Here's how the part is built. I have some questions about the finished solid (model axes, mm). A direction names the side the tool comes from. Round coordinates to 2 decimals unless told otherwise and drop trailing zeros. Write each loop counter-clockwise with the first axis right and the second up, starting at its lowest first coordinate (ties: lowest second). Pieces come first, ordered by that corner, then holes. Notation, with made-up numbers: (-39, 30) -> (-22, 30) arc R6 ccw to (-22, 41) -> close; hole circle Ø7 at (85, -26.75). An arc over 180 degrees is marked (long way). Put each result on its own line as item: value. Start each with the question number.
1) If I drill on line 1 along X through (y, z) = (14.75, -7.5); line 2 along Z through (x, y) = (8.5, 11.5); line 3 along Z through (x, y) = (14, 6), over which ranges is the centre line in solid material (lowest first)? Write a range as [from, to].
2) I want a section at A-A, the plane z = -7. List the corners of the cut face in (x, y) for me.
3) We'd pull the mould along Z, two halves only. Please class faces 1 (the conical face through (3.18, 16.99, -3.24)), 2 (the conical face through (37.436, 16.986, -80.218)), 3 (the flat face through (0.947, 16.986, -40.345)), 4 (the conical face through (35.82, 16.99, -78.51)): released by +Z, released by -Z, zero draft, split by the parting line, or undercut.
4) I want a section at D-D, the plane y = 11. List the corners of the cut face in (x, z) for me, then the cut area to 4 significant figures.
5) Will these pins go through, and if not, where does the flat tip stop? P1, Ø0.9, axis at y = 11, z = -2, coming from the -X side; P2, Ø1.5, axis at x = 21, z = -2, coming from the +Y side; P3, Ø2, axis at y = 16.5, z = -79.5, coming from the +X side; P4, Ø3.5, axis at x = 8.5, z = -54, coming from the +Y side.
6) I want a section at C-C, the plane y = 15.25. List the corners of the cut face in (x, z) for me, then the cut area to 3 significant figures.
7) I want a section at B-B, the plane x = 30. List the corners of the cut face in (y, z) for me.
8) Which directions (+Z, -Z, +X, -X, +Y, -Y) give clear straight access to the entire face, cutting with the end or side of a thin tool? Please do faces 5 (the cylindrical face through (38.1, 8.6, -0.86)), 6 (the flat face through (11, 11, -1)), 7 (the flat face through (19, 14, -80)), 8 (the conical face through (37.5, 17, -1.6)), 9 (the flat face through (8.465, 16.986, -2.053)).
from build123d import *

# Parameters (mm, degrees)
SKETCH1_W                 = 39
SKETCH1_H                 = 81.75
BOSS_EXTRUDE1_DEPTH       = 3
SKETCH2_W                 = 39
SKETCH2_H                 = 81.75
SKETCH2_W_2               = 33
SKETCH2_H_2               = 75.75
BOSS_EXTRUDE2_DEPTH       = 15
SKETCH4_W                 = 17
SKETCH4_H                 = 3
CUT_EXTRUDE1_DEPTH        = 14
SKETCH4_3_W               = 12
SKETCH4_3_H               = 3
CUT_EXTRUDE2_DEPTH        = 4
FILLET1_R                 = 3
STANDOFFS1_GROOVE_DEPTH   = 2
STANDOFFS1_GROOVE_DRAFT   = -3
STANDOFFS1_GROOVE_2_DEPTH = 2
STANDOFFS1_GROOVE_2_DRAFT = -3
STANDOFFS2_GROOVE_DEPTH   = 2
STANDOFFS2_GROOVE_DRAFT   = -3
STANDOFFS2_GROOVE_2_DEPTH = 2
STANDOFFS2_GROOVE_2_DRAFT = -3
FILLET2_R                 = 2
CHAMFER1_SIZE             = 1


# Read off the part's stored shape, not the designer's step: Standoffs1-Groove, Standoffs2-Groove
with BuildPart() as part:
    # Sketch1 → Boss-Extrude1 (new body)
    with BuildSketch(Plane(origin=(0, 0, 0), x_dir=(1, 0, 0), z_dir=(0, 1, 0))):
        with Locations((19.5, 40.875)):
            Rectangle(SKETCH1_W, SKETCH1_H)
    extrude(amount=BOSS_EXTRUDE1_DEPTH)

    # Sketch2 → Boss-Extrude2 (add)
    with BuildSketch(Plane(origin=(0, 3, 0), x_dir=(1, 0, 0), z_dir=(0, 1, 0))):
        with Locations((19.5, 40.875)):
            Rectangle(SKETCH2_W, SKETCH2_H)
        with Locations((19.5, 40.875)):
            Rectangle(SKETCH2_W_2, SKETCH2_H_2, mode=Mode.SUBTRACT)
    extrude(amount=BOSS_EXTRUDE2_DEPTH)

    # Sketch4 → Cut-Extrude1 (cut)
    with BuildSketch(Plane(origin=(0, 18, 0), x_dir=(1, 0, 0), z_dir=(0, 1, 0))):
        with Locations((19.5, 1.5)):
            Rectangle(SKETCH4_W, SKETCH4_H)
    extrude(amount=-CUT_EXTRUDE1_DEPTH, mode=Mode.SUBTRACT)

    # Sketch4<3> → Cut-Extrude2 (cut)
    with BuildSketch(Plane(origin=(0, 18, 0), x_dir=(1, 0, 0), z_dir=(0, 1, 0))):
        with Locations((19.5, 80.25)):
            Rectangle(SKETCH4_3_W, SKETCH4_3_H)
    extrude(amount=-CUT_EXTRUDE2_DEPTH, mode=Mode.SUBTRACT)

    # Fillet1
    fillet1_edges = [part.edges().sort_by_distance(p)[0] for p in [
        (3, 10.5, -78.75),
        (3, 10.5, -3),
        (36, 10.5, -3),
        (36, 10.5, -78.75),
        (0, 9, -81.75),
        (39, 9, -81.75),
        (39, 9, 0),
        (0, 9, 0),
    ]]
    fillet(fillet1_edges, radius=FILLET1_R)


with BuildPart() as standoffs1_groove_tool:
    # Standoffs1-Groove outline → Standoffs1-Groove (with draft: the straight prism first)
    with BuildSketch(Plane(origin=(0, 16, 0), x_dir=(1, 0, 0), z_dir=(0, 1, 0))):
        with BuildLine():
            Line((11, 0.895184441), (3, 0.895184441))
            ThreePointArc((3, 0.895184441), (1.511670645, 1.511670645), (0.895184441, 3))
            Line((0.895184441, 3), (0.895184441, 78.75))
            ThreePointArc((0.895184441, 78.75), (1.511670645, 80.238329355), (3, 80.854815559))
            Line((3, 80.854815559), (13.5, 80.854815559))
            Line((13.5, 80.854815559), (13.5, 81.75))
            Line((13.5, 81.75), (3, 81.75))
            ThreePointArc((3, 81.75), (0.878679656, 80.871320344), (0, 78.75))
            Line((0, 78.75), (0, 3))
            ThreePointArc((0, 3), (0.878679656, 0.878679656), (3, 0))
            Line((3, 0), (11, 0))
            Line((11, 0), (11, 0.895184441))
        make_face()
    extrude(amount=STANDOFFS1_GROOVE_DEPTH)
    # Standoffs1-Groove: the draft: its side faces are tilted about the plane it starts from
    standoffs1_groove_sides = [standoffs1_groove_tool.faces().sort_by_distance(p)[0] for p in [
        (7, 17, -0.895184441),
        (1.511670645, 17, -1.511670645),
        (0.895184441, 17, -40.875),
        (1.511670645, 17, -80.238329355),
        (8.25, 17, -80.854815559),
        (13.5, 17, -81.30240778),
        (8.25, 17, -81.75),
        (0.878679656, 17, -80.871320344),
        (0, 17, -40.875),
        (0.878679656, 17, -0.878679656),
        (7, 17, 0),
        (11, 17, -0.447592221),
    ]]
    draft(standoffs1_groove_sides, Plane(origin=(0, 16, 0), x_dir=(1, 0, 0), z_dir=(0, 1, 0)), STANDOFFS1_GROOVE_DRAFT)


with BuildPart() as part_1:
    add(part.part)

    # Standoffs1-Groove: cut by standoffs1_groove_tool
    add(standoffs1_groove_tool.part, mode=Mode.SUBTRACT)


with BuildPart() as standoffs1_groove_2_tool:
    # Standoffs1-Groove 2 outline → Standoffs1-Groove 2 (with draft: the straight prism first)
    with BuildSketch(Plane(origin=(0, 16, 0), x_dir=(1, 0, 0), z_dir=(0, 1, 0))):
        with BuildLine():
            Line((11, 3), (6, 3))
            ThreePointArc((6, 3), (3.878679656, 3.878679656), (3, 6))
            Line((3, 6), (3, 75.75))
            ThreePointArc((3, 75.75), (3.878679656, 77.871320344), (6, 78.75))
            Line((6, 78.75), (13.5, 78.75))
            Line((13.5, 78.75), (13.5, 79.645184441))
            Line((13.5, 79.645184441), (6, 79.645184441))
            ThreePointArc((6, 79.645184441), (3.245688667, 78.504311333), (2.104815559, 75.75))
            Line((2.104815559, 75.75), (2.104815559, 6))
            ThreePointArc((2.104815559, 6), (3.245688667, 3.245688667), (6, 2.104815559))
            Line((6, 2.104815559), (11, 2.104815559))
            Line((11, 2.104815559), (11, 3))
        make_face()
    extrude(amount=STANDOFFS1_GROOVE_2_DEPTH)
    # Standoffs1-Groove 2: the draft: its side faces are tilted about the plane it starts from
    standoffs1_groove_2_sides = [standoffs1_groove_2_tool.faces().sort_by_distance(p)[0] for p in [
        (3.245688667, 17, -78.504311333),
        (2.104815559, 17, -40.875),
        (3.245688667, 17, -3.245688667),
        (8.5, 17, -2.104815559),
        (11, 17, -2.552407779),
        (8.5, 17, -3),
        (3.878679656, 17, -3.878679656),
        (3, 17, -40.875),
        (3.878679656, 17, -77.871320344),
        (9.75, 17, -78.75),
        (13.5, 17, -79.19759222),
        (9.75, 17, -79.645184441),
    ]]
    draft(standoffs1_groove_2_sides, Plane(origin=(0, 16, 0), x_dir=(1, 0, 0), z_dir=(0, 1, 0)), STANDOFFS1_GROOVE_2_DRAFT)


with BuildPart() as part_2:
    add(part_1.part)

    # Standoffs1-Groove 2: cut by standoffs1_groove_2_tool
    add(standoffs1_groove_2_tool.part, mode=Mode.SUBTRACT)


with BuildPart() as standoffs2_groove_tool:
    # Standoffs2-Groove outline → Standoffs2-Groove (with draft: the straight prism first)
    with BuildSketch(Plane(origin=(0, 16, 0), x_dir=(1, 0, 0), z_dir=(0, 1, 0))):
        with BuildLine():
            Line((25.5, 81.75), (25.5, 80.854815559))
            Line((25.5, 80.854815559), (36, 80.854815559))
            ThreePointArc((36, 80.854815559), (37.488329355, 80.238329355), (38.104815559, 78.75))
            Line((38.104815559, 78.75), (38.104815559, 3))
            ThreePointArc((38.104815559, 3), (37.488329355, 1.511670645), (36, 0.895184441))
            Line((36, 0.895184441), (28, 0.895184441))
            Line((28, 0.895184441), (28, 0))
            Line((28, 0), (36, 0))
            ThreePointArc((36, 0), (38.121320344, 0.878679656), (39, 3))
            Line((39, 3), (39, 78.75))
            ThreePointArc((39, 78.75), (38.121320344, 80.871320344), (36, 81.75))
            Line((36, 81.75), (25.5, 81.75))
        make_face()
    extrude(amount=STANDOFFS2_GROOVE_DEPTH)
    # Standoffs2-Groove: the draft: its side faces are tilted about the plane it starts from
    standoffs2_groove_sides = [standoffs2_groove_tool.faces().sort_by_distance(p)[0] for p in [
        (25.5, 17, -81.30240778),
        (30.75, 17, -80.854815559),
        (37.488329355, 17, -80.238329355),
        (38.104815559, 17, -40.875),
        (37.488329355, 17, -1.511670645),
        (32, 17, -0.895184441),
        (28, 17, -0.447592221),
        (32, 17, 0),
        (38.121320344, 17, -0.878679656),
        (39, 17, -40.875),
        (38.121320344, 17, -80.871320344),
        (30.75, 17, -81.75),
    ]]
    draft(standoffs2_groove_sides, Plane(origin=(0, 16, 0), x_dir=(1, 0, 0), z_dir=(0, 1, 0)), STANDOFFS2_GROOVE_DRAFT)


with BuildPart() as part_3:
    add(part_2.part)

    # Standoffs2-Groove: cut by standoffs2_groove_tool
    add(standoffs2_groove_tool.part, mode=Mode.SUBTRACT)


with BuildPart() as standoffs2_groove_2_tool:
    # Standoffs2-Groove 2 outline → Standoffs2-Groove 2 (with draft: the straight prism first)
    with BuildSketch(Plane(origin=(0, 16, 0), x_dir=(1, 0, 0), z_dir=(0, 1, 0))):
        with BuildLine():
            Line((28, 3), (28, 2.104815559))
            Line((28, 2.104815559), (33, 2.104815559))
            ThreePointArc((33, 2.104815559), (35.754311333, 3.245688667), (36.895184441, 6))
            Line((36.895184441, 6), (36.895184441, 75.75))
            ThreePointArc((36.895184441, 75.75), (35.754311333, 78.504311333), (33, 79.645184441))
            Line((33, 79.645184441), (25.5, 79.645184441))
            Line((25.5, 79.645184441), (25.5, 78.75))
            Line((25.5, 78.75), (33, 78.75))
            ThreePointArc((33, 78.75), (35.121320344, 77.871320344), (36, 75.75))
            Line((36, 75.75), (36, 6))
            ThreePointArc((36, 6), (35.121320344, 3.878679656), (33, 3))
            Line((33, 3), (28, 3))
        make_face()
    extrude(amount=STANDOFFS2_GROOVE_2_DEPTH)
    # Standoffs2-Groove 2: the draft: its side faces are tilted about the plane it starts from
    standoffs2_groove_2_sides = [standoffs2_groove_2_tool.faces().sort_by_distance(p)[0] for p in [
        (30.5, 17, -3),
        (28, 17, -2.552407779),
        (30.5, 17, -2.104815559),
        (35.754311333, 17, -3.245688667),
        (36.895184441, 17, -40.875),
        (35.754311333, 17, -78.504311333),
        (29.25, 17, -79.645184441),
        (25.5, 17, -79.19759222),
        (29.25, 17, -78.75),
        (35.121320344, 17, -77.871320344),
        (36, 17, -40.875),
        (35.121320344, 17, -3.878679656),
    ]]
    draft(standoffs2_groove_2_sides, Plane(origin=(0, 16, 0), x_dir=(1, 0, 0), z_dir=(0, 1, 0)), STANDOFFS2_GROOVE_2_DRAFT)


with BuildPart() as part_4:
    add(part_3.part)

    # Standoffs2-Groove 2: cut by standoffs2_groove_2_tool
    add(standoffs2_groove_2_tool.part, mode=Mode.SUBTRACT)

    # Fillet2
    fillet2_edges = [part_4.edges().sort_by_distance(p)[0] for p in [
        (25.5, 14, -80.25),
        (13.5, 14, -80.25),
        (11, 4, -1.5),
        (28, 4, -1.5),
    ]]
    fillet(fillet2_edges, radius=FILLET2_R - 0.0001)  # a hair under: the kernel refuses the full size

    # Chamfer1
    chamfer1_edges = [part_4.edges().sort_by_distance(p)[0] for p in [
        (19.5, 0, 0),
        (0, 0, -40.875),
        (19.5, 0, -81.75),
        (39, 0, -40.875),
        (38.121320344, 0, -0.878679656),
        (0.878679656, 0, -80.871320344),
        (38.121320344, 0, -80.871320344),
        (0.878679656, 0, -0.878679656),
    ]]
    chamfer(chamfer1_edges, length=CHAMFER1_SIZE)


solid = part_4.part
Findings:
1. line 1: x = [0, 3], [36, 39]
1. line 2: z = [-81.75, -78.75], [-3, 0]
1. line 3: z = [-81.75, -78.75]
2. outline: (0, 1) -> (1, 0) -> (38, 0) -> (39, 1) -> (39, 16) -> (38.1, 16) -> (38, 18) -> (37, 18) -> (36.9, 16) -> (36, 16) -> (36, 3) -> (3, 3) -> (3, 16) -> (2.1, 16) -> (2, 18) -> (1, 18) -> (0.9, 16) -> (0, 16) -> close
3. face 1: undercut
3. face 2: released by -Z
3. face 3: zero draft
3. face 4: undercut
4. outline: (0, -78.75) arc R3 ccw to (3, -81.75) -> (36, -81.75) arc R3 ccw to (39, -78.75) -> (39, -3) arc R3 ccw to (36, 0) -> (28, 0) -> (28, -3) -> (33, -3) arc R3 cw to (36, -6) -> (36, -75.75) arc R3 cw to (33, -78.75) -> (6, -78.75) arc R3 cw to (3, -75.75) -> (3, -6) arc R3 cw to (6, -3) -> (11, -3) -> (11, 0) -> (3, 0) arc R3 ccw to (0, -3) -> close
4. area: 637.5 mm2
5. P1: stops at x = 0.05
5. P2: stops at y = 4
5. P3: stops at x = 39
5. P4: stops at y = 3
6. outline: (0, -78.75) arc R3 ccw to (3, -81.75) -> (13.65, -81.75) -> (13.65, -78.75) -> (6, -78.75) arc R3 cw to (3, -75.75) -> (3, -6) arc R3 cw to (6, -3) -> (11, -3) -> (11, 0) -> (3, 0) arc R3 ccw to (0, -3) -> close; (25.35, -81.75) -> (36, -81.75) arc R3 ccw to (39, -78.75) -> (39, -3) arc R3 ccw to (36, 0) -> (28, 0) -> (28, -3) -> (33, -3) arc R3 cw to (36, -6) -> (36, -75.75) arc R3 cw to (33, -78.75) -> (25.35, -78.75) -> close
6. area: 602 mm2
7. outline: (0, -80.75) -> (1, -81.75) -> (16, -81.75) -> (16, -80.85) -> (18, -80.75) -> (18, -79.75) -> (16, -79.65) -> (16, -78.75) -> (3, -78.75) -> (3, -3) -> (16, -3) -> (16, -2.1) -> (18, -2) -> (18, -1) -> (16, -0.9) -> (16, 0) -> (1, 0) -> (0, -1) -> close
8. face 5: +Z, +X, +Y, -Y
8. face 6: +Z, +Y
8. face 7: +Z, -Z, +Y
8. face 8: +Z, +X, +Y
8. face 9: +Y
